from build123d import *

# Parameters (mm, degrees)
F0_W     = 150
F0_H     = 50
F1_DEPTH = 50
F2_R     = 2.5
F3_DEPTH = 50
F4_R     = 10
F5_DEPTH = 100


with BuildPart() as f1:
    # F0 (on Front) → F1 (new body)
    with BuildSketch(Plane.XZ):
        with Locations((25, 25)):
            Rectangle(F0_W, F0_H)
    extrude(amount=F1_DEPTH)

    # F2 (on Front) → F3 (cut)
    with BuildSketch(Plane.XZ):
        with Locations((-30, 30)):
            Circle(F2_R)
    extrude(amount=F3_DEPTH, mode=Mode.SUBTRACT)

    # F4 (on face) → F5 (cut)
    with BuildSketch(Plane(origin=(-50, 0, 0), x_dir=(0, -1, 0), z_dir=(-1, 0, 0))):
        with Locations((25, 30)):
            Circle(F4_R)
    extrude(amount=-F5_DEPTH, mode=Mode.SUBTRACT)


solid = f1.part
The model under review builds one solid part; all positions refer to its coordinate system, in mm. A direction names the side the tool comes from. Give positions to 0.01 mm unless a question says otherwise; leave off trailing zeros. Loops run counter-clockwise (first coordinate to the right, second up) from the corner with the lowest first, then second, coordinate; pieces in that order, holes last. Notation, with made-up numbers: (62.5, 67.5) -> (104.5, 67.5) arc R26 cw to (104.5, 105.5) -> close; hole circle Ø11 at (-7.5, 21). An arc over 180 degrees is marked (long way). Answer as a JSON object with one key per item and string values. Group by question number.
Q1. Take a section at A-A (x = -30). Write out the cut boundary in (y, z).
Q2. Tool access review of faces 1 (the flat face through (24, 0, 25)), 2 (the cylindrical face through (-0.7, -29.614, 21.128)): name each direction out of +Z, -Z, +X, -X, +Y, -Y from which nothing blocks a thin tool from reaching the whole face with its end or side.
Q3. Wall thickness on line 1 along Y through (x, z) = (10, 32.5); line 2 along Z through (x, y) = (-30, -44.5); line 3 along Z through (x, y) = (-39, -25.5): over which ranges is each line inside the solid? List them lowest first.
Q4. Draft analysis for pull direction Z (two halves, no side actions). For faces 3 (the flat face through (50, -25, 30)), 4 (the flat face through (24, -25, 50)), 5 (the flat face through (24, -25, 0)), state which applies: pulls with the +Z half, pulls with the -Z half, needs draft (parallel to the pull), parting line crosses it, or undercut.
Q5. Take a section at C-C (x = 6). Write out the cut boundary in (y, z), plus the area to 3 significant figures.
Q6. Take a section at D-D (y = -25). Write out the cut boundary in (x, z), plus the area to 3 significant figures.
Q7. Insertion check: pin 1 (6 mm diameter, centred on y = -20.5, z = 32, fed in from -X); pin 2 (3 mm diameter, centred on x = -30, z = 30, fed in from +Y). Each pin has a flat end and moves straight along its axis. Give the tip position at first contact, or say it passes through.
Q8. Take a section at B-B (z = 30). Write out the cut boundary in (x, y).
Answer below:
{
 "1": {"outline": "(-50, 0) -> (0, 0) -> (0, 27.5) -> (-15.32, 27.5) arc R10 cw to (-34.68, 27.5) -> (-50, 27.5) -> close; (-50, 32.5) -> (-34.68, 32.5) arc R10 cw to (-15.32, 32.5) -> (0, 32.5) -> (0, 50) -> (-50, 50) -> close"},
 "2": {"face 1": "+Z, -Z, +X, -X, +Y", "face 2": "-X"},
 "3": {"line 1": "y = -50 to -34.68, -15.32 to 0", "line 2": "z = 0 to 27.5, 32.5 to 50", "line 3": "z = 0 to 20.01, 39.99 to 50"},
 "4": {"face 3": "undercut", "face 4": "pulls with the +Z half", "face 5": "pulls with the -Z half"},
 "5": {"outline": "(-50, 0) -> (0, 0) -> (0, 50) -> (-50, 50) -> close; hole circle Ø20 at (-25, 30)", "area": "2,190 mm2"},
 "6": {"outline": "(-50, 0) -> (100, 0) -> (100, 50) -> (-50, 50) -> (-50, 40) -> (50, 40) -> (50, 20) -> (-50, 20) -> close", "area": "5,500 mm2"},
 "7": {"pin 1": "stops at x = 50", "pin 2": "passes through"},
 "8": {"outline": "(-50, -50) -> (-32.5, -50) -> (-32.5, -35) -> (-50, -35) -> close; (-50, -15) -> (-32.5, -15) -> (-32.5, 0) -> (-50, 0) -> close; (-27.5, -50) -> (100, -50) -> (100, 0) -> (-27.5, 0) -> (-27.5, -15) -> (50, -15) -> (50, -35) -> (-27.5, -35) -> close"}
}
